Autodesk Inventor part; units mm, degrees
ref_plane "bspg_r2_XY" through (28.5, 4.5, 0) normal (1, 0, 0) x (0, 0, -1)
ref_plane "bspg_r2_YZ" through (28.5, 4.5, 0) normal (0, 0, -1) x (0, 1, 0)
ref_plane "bspg_r2_ZX" through (28.5, 4.5, 0) normal (0, 1, 0) x (1, 0, 0)
sketch "Sketch_1" plane through (0, 0, 0) normal (1, 0, 0) x (0, 1, 0)
  line L0 (4.5, 4.8) -> (2.15, 4.8)
  arc A0 (2.15, 4.8) -> (0, 2.65) centre (2.15, 2.65) ccw
  line L1 (0, 2.65) -> (0, -2.65)
  arc A1 (0, -2.65) -> (2.15, -4.8) centre (2.15, -2.65) ccw
  line L2 (2.15, -4.8) -> (4.5, -4.8)
  line L3 (4.5, -4.8) -> (4.5, -3.6)
  line L4 (4.5, -3.6) -> (2, -3.6)
  arc A2 (1.2, -2.8) -> (2, -3.6) centre (2, -2.8) ccw
  line L5 (1.2, -2.8) -> (1.2, 2.8)
  arc A3 (2, 3.6) -> (1.2, 2.8) centre (2, 2.8) ccw
  line L6 (2, 3.6) -> (4.5, 3.6)
  line L7 (4.5, 3.6) -> (4.5, 4.8)
extrude "Extrusion1" add sketch "Sketch_1" along normal blind 57
sketch "Sketch_2" plane through (8.5, 0, 0) normal (1, 0, 0) x (0, 0, -1)
  line L0 (0, 0) -> (0, 1.2)
  line L1 (0, 1.2) -> (1.5, 1.2)
  line L2 (1.5, 1.2) -> (1.2295, 0.9295)
  line L3 (1.2295, 0.9295) -> (1.2295, 0.2705)
  line L4 (1.2295, 0.2705) -> (1.5, 0)
  line L5 (1.5, 0) -> (0, 0)
  line L6 (0, 0) -> (0, 1.2)
revolve "Revolution1" cut sketch "Sketch_2" angle 360 about axis through (8.5, 0, 0) along (0, -1, 0)
thread "Thread1"
sketch "Sketch_3" plane through (48.5, 0, 0) normal (1, 0, 0) x (0, 0, -1)
  line L0 (0, 0) -> (0, 1.2)
  line L1 (0, 1.2) -> (1.5, 1.2)
  line L2 (1.5, 1.2) -> (1.2295, 0.9295)
  line L3 (1.2295, 0.9295) -> (1.2295, 0.2705)
  line L4 (1.2295, 0.2705) -> (1.5, 0)
  line L5 (1.5, 0) -> (0, 0)
  line L6 (0, 0) -> (0, 1.2)
revolve "Revolution2" cut sketch "Sketch_3" angle 360 about axis through (48.5, 0, 0) along (0, -1, 0)
thread "Thread2"
sketch "Sketch4" plane through (0, 0, -2.65) normal (0, -1, 0) x (1, 0, 0)
  point P0 (20.95, 2.65)
hole "Hole1" at (20.95, 0, 0) direction (0, 1, 0) diameter 1.8 depth 1.2
sketch "Sketch5" plane through (0, 0, -2.65) normal (0, -1, 0) x (1, 0, 0)
  point P0 (36.05, 2.65)
hole "Hole2" at (36.05, 0, 0) direction (0, 1, 0) diameter 1.8 depth 1.2
sketch "Sketch_8" plane through (28.5, 0, 0) normal (1, 0, 0) x (0, 0, -1)
  arc A0 (5.1667, 4.4667) -> (5.1667, 2.2667) centre (5.1667, 3.3667) ccw
  line L0 (5.1667, 2.2667) -> (5.1667, 4.4667)
extrude "Extrusion2" cut sketch "Sketch_8" along normal mid plane 36
sketch "Sketch_10" plane through (28.5, 0, 0) normal (1, 0, 0) x (0, 0, -1)
  arc A0 (-5.1667, 2.2667) -> (-5.1667, 4.4667) centre (-5.1667, 3.3667) ccw
  line L0 (-5.1667, 4.4667) -> (-5.1667, 2.2667)
extrude "Extrusion3" cut sketch "Sketch_10" along normal mid plane 36
ref_plane "bspg_r2_XY" through (28.5, 4.5, 0) normal (1, 0, 0) x (0, 0, -1)
ref_plane "bspg_r2_YZ" through (28.5, 4.5, 0) normal (0, 0, -1) x (0, 1, 0)
ref_plane "bspg_r2_ZX" through (28.5, 4.5, 0) normal (0, 1, 0) x (1, 0, 0)
properties part number "BSPG1560 Rail"
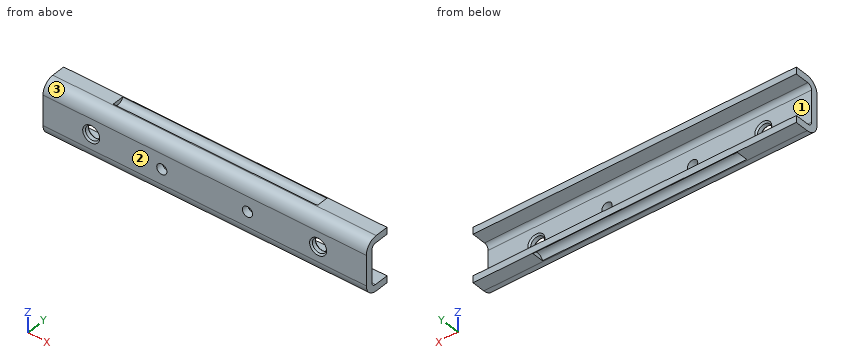
Geometry: final body of the model. Coordinates: model frame, mm. Face numbers are marked on the shaded views. Round coordinates to 2 decimals unless told otherwise and drop trailing zeros. Order: outer loops, then holes, each group sorted by start corner. A loop starts at its lowest first (then second) coordinate and runs counter-clockwise, first axis right, second up.
Q1. Section C-C, the plane y = 3. Output: boundary loops of the cut face in (x, z).
Result sheet:
outline: (0, -4.8) - (10.5, -4.8) - (10.5, -4.13) - (46.5, -4.13) - (46.5, -4.8) - (57, -4.8) - (57, -3.6) - (0, -3.6) - close; (0, 3.6) - (57, 3.6) - (57, 4.8) - (46.5, 4.8) - (46.5, 4.13) - (10.5, 4.13) - (10.5, 4.8) - (0, 4.8) - close
Q2. Section D-D, the plane x = 48.5. Output: boundary loops of the cut face in (y, z), and give its area (3 significant figures).
Result sheet:
outline: (0, -2.65) arc R2.15 ccw to (2.15, -4.8) - (4.5, -4.8) - (4.5, -3.6) - (2, -3.6) arc R0.8 cw to (1.2, -2.8) - (1.2, -1.5) - (0.93, -1.23) - (0.27, -1.23) - (0, -1.5) - close; (0, 1.5) - (0.27, 1.23) - (0.93, 1.23) - (1.2, 1.5) - (1.2, 2.8) arc R0.8 cw to (2, 3.6) - (4.5, 3.6) - (4.5, 4.8) - (2.15, 4.8) arc R2.15 ccw to (0, 2.65) - close
area: 14.6 mm2
Q3. Pin query (flat end, axial travel): pin 1 (1 mm diameter, centred on x = 47, y = 1.5, fed in from -Z); pin 2 (4.5 mm diameter, centred on x = 31, z = 1, fed in from +Y); pin 3 (1.2 mm diameter, centred on x = 22, y = 3.5, fed in from +Z); pin 4 (1 mm diameter, centred on y = 2, z = 2.5, fed in from +X). Return the tip coordinate at first contact, or that it passes through.
Result sheet:
pin 1: stops at z = -4.79
pin 2: stops at y = 1.34
pin 3: stops at z = 4.35
pin 4: passes through
Q4. Section A-A, the plane x = 36.05. Output: boundary loops of the cut face in (y, z), and give its area (3 significant figures).
Result sheet:
outline: (0, -2.65) arc R2.15 ccw to (2.15, -4.8) - (2.33, -4.8) arc R1.1 cw to (4.4, -4.8) - (4.5, -4.8) - (4.5, -3.6) - (2, -3.6) arc R0.8 cw to (1.2, -2.8) - (1.2, -0.9) - (0, -0.9) - close; (0, 0.9) - (1.2, 0.9) - (1.2, 2.8) arc R0.8 cw to (2, 3.6) - (4.5, 3.6) - (4.5, 4.8) - (4.4, 4.8) arc R1.1 cw to (2.33, 4.8) - (2.15, 4.8) arc R2.15 ccw to (0, 2.65) - close
area: 13.4 mm2
Q5. Section B-B, the plane z = 0. Output: boundary loops of the cut face in (x, y), and give its area (3 significant figures).
Result sheet:
outline: (0, 0) - (7, 0) - (7.27, 0.27) - (7.27, 0.93) - (7, 1.2) - (0, 1.2) - close; (9.73, 0.27) - (10, 0) - (20.05, 0) - (20.05, 1.2) - (10, 1.2) - (9.73, 0.93) - close; (21.85, 0) - (35.15, 0) - (35.15, 1.2) - (21.85, 1.2) - close; (36.95, 0) - (47, 0) - (47.27, 0.27) - (47.27, 0.93) - (47, 1.2) - (36.95, 1.2) - close; (49.73, 0.27) - (50, 0) - (57, 0) - (57, 1.2) - (50, 1.2) - (49.73, 0.93) - close
area: 57.9 mm2
Q6. Material intervals for probe 1 along X at (y, z) = (0.55, 0); probe 2 along Z at (x, y) = (48, 2.15); probe 3 along Z at (x, y) = (40, 4.05), sorted ascending.
Result sheet:
probe 1: x = 0 to 7.27, 9.73 to 20.05, 21.85 to 35.15, 36.95 to 47.27, 49.73 to 57
probe 2: z = -4.8 to -3.6, 3.6 to 4.8
probe 3: z = -4.3 to -3.6, 3.6 to 4.3
Q7. Mould query, pull axis Z, two halves, no side actions, for the marked faces 1, 2 and 3. Classes: released by +Z, released by -Z, zero draft, split by the parting line, or undercut.
Result sheet:
face 1: undercut
face 2: zero draft
face 3: released by +Z
